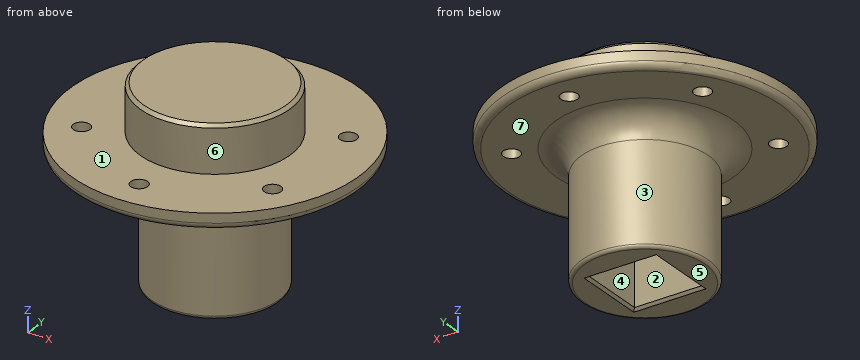
```python
from build123d import *

# Parameters (mm, degrees)
SKETCH1_R           = 20
BOSS_EXTRUDE1_DEPTH = 40
SKETCH2_W           = 21.283914114
SKETCH2_H           = 21.283914114
CUT_EXTRUDE1_DEPTH  = 15
CHAMFER1_SIZE       = 0.8
SKETCH3_R           = 45
BOSS_EXTRUDE2_DEPTH = 5
SKETCH4_R           = 23.5
BOSS_EXTRUDE3_DEPTH = 14.7
CHAMFER2_SIZE       = 1
FILLET1_R           = 2
FILLET2_R           = 8
SKETCH5_R           = 2.65
CUT_EXTRUDE2_DEPTH  = 78.942286398
CIRPATTERN1_COUNT   = 6
FILLET3_R           = 1


with BuildPart() as part:
    # Sketch1 → Boss-Extrude1 (new body)
    with BuildSketch(Plane.XY):
        Circle(SKETCH1_R)
    extrude(amount=BOSS_EXTRUDE1_DEPTH)

    # Sketch2 → Cut-Extrude1 (cut)
    with BuildSketch(Plane(origin=(0, 0, 0), x_dir=(-1, 0, 0), z_dir=(0, 0, -1))):
        Rectangle(SKETCH2_W, SKETCH2_H)
    extrude(amount=-CUT_EXTRUDE1_DEPTH, mode=Mode.SUBTRACT)

    # Chamfer1
    chamfer1_edges = [part.edges().sort_by_distance(p)[0] for p in [
        (0, -10.641957057, 0),
        (-10.641957057, 0, 0),
        (0, 10.641957057, 0),
        (10.641957057, 0, 0),
    ]]
    chamfer(chamfer1_edges, length=CHAMFER1_SIZE)

    # Sketch3 → Boss-Extrude2 (add)
    with BuildSketch(Plane.XY.offset(40)):
        Circle(SKETCH3_R)
    extrude(amount=BOSS_EXTRUDE2_DEPTH)

    # Sketch4 → Boss-Extrude3 (add)
    with BuildSketch(Plane.XY.offset(45)):
        Circle(SKETCH4_R)
    extrude(amount=BOSS_EXTRUDE3_DEPTH)

    # Chamfer2
    chamfer2_edges = [part.edges().sort_by_distance(p)[0] for p in [
        (-23.5, 0, 59.7),
    ]]
    chamfer(chamfer2_edges, length=CHAMFER2_SIZE)

    # Fillet1
    fillet1_edges = [part.edges().sort_by_distance(p)[0] for p in [
        (-45, 0, 40),
    ]]
    fillet(fillet1_edges, radius=FILLET1_R)

    # Fillet2
    fillet2_edges = [part.edges().sort_by_distance(p)[0] for p in [
        (-20, 0, 40),
    ]]
    fillet(fillet2_edges, radius=FILLET2_R)

    # Sketch5 → Cut-Extrude2 (cut, through all)
    with BuildSketch(Plane.XY.offset(45)):
        with Locations((0, 35)):
            Circle(SKETCH5_R)
    cut_extrude2 = extrude(amount=-CUT_EXTRUDE2_DEPTH, mode=Mode.SUBTRACT)

    # CirPattern1: Cut-Extrude2 ×6 about axis
    cirpattern1_axis = Axis((0, 0, 0), (0, 0, 1))
    for i in range(1, CIRPATTERN1_COUNT):
        add(cut_extrude2.rotate(cirpattern1_axis, i * 360 / CIRPATTERN1_COUNT), mode=Mode.SUBTRACT)

    # Fillet3
    fillet3_edges = [part.edges().sort_by_distance(p)[0] for p in [
        (-20, 0, 0),
    ]]
    fillet(fillet3_edges, radius=FILLET3_R)


solid = part.part
```
Geometry: final body of the model. Coordinates: model frame, mm. Face numbers are marked on the shaded views. A direction names the side the tool comes from. Round coordinates to 2 decimals unless told otherwise and drop trailing zeros. Write each loop counter-clockwise with the first axis right and the second up, starting at its lowest first coordinate (ties: lowest second). Pieces come first, ordered by that corner, then holes. Notation, with made-up numbers: (81, 38) -> (109, 38) arc R26 cw to (109, 65) -> close; hole circle Ø5 at (-19.5, -14). An arc over 180 degrees is marked (long way). Use CSV: the item, a comma, the result in double quotes. Start each with the question number.
Q1. Section A-A (x = 0). Give the number of separate pieces and of enclosed holes in the cut face, plus the area to 3 significant figures.
Q2. Line query: L1, parallel to Y at x = 0, z = 43.4; L2, parallel to Z at x = 9.5, y = 7; L3, parallel to Y at x = 0.5, z = 57.5. Output: solid intervals per line, ascending.
Q3. Section C-C (y = 0). Return loops of the section in (x, z), plus the area to 3 significant figures.
Q4. Section B-B (z = 10). Return loops of the section in (x, y), plus the area to 3 significant figures.
Q5. Reachability of the marked faces 5, 6 and 7 from +Z, -Z, +X, -X, +Y, -Y: full face, straight path, thin tool, end or side. Return the list, or none.
Q6. First-contact query: pin 1 Ø4.5 at (y, z) = (2, 9.5) entering from +X; pin 2 Ø11.5 at (x, z) = (-4.5, 10) entering from -Y; pin 3 Ø6 at (x, y) = (30.31, -17.5) entering from +Z. Flat tips, straight axial feed; report the tip coordinate or a pass-through.
Q7. Pull-direction query (Y, two-part tool) for the marked faces 1, 2, 3 and 4; classes: pulls with the +Y half, pulls with the -Y half, needs draft (parallel to the pull), parting line crosses it, or undercut.
Result sheet:
1,separate pieces,"3"
1,enclosed holes,"0"
1,area,"2,390 mm²"
2,L1,"-45 to -37.65, -32.35 to 32.35, 37.65 to 45"
2,L2,"15 to 59.7"
2,L3,"-23.49 to 23.49"
3,outline,"(-45, 42) arc R2 ccw to (-43, 40) -> (-28, 40) arc R8 cw to (-20, 32) -> (-20, 1) arc R1 ccw to (-19, 0) -> (-11.44, 0) -> (-10.64, 0.8) -> (-10.64, 15) -> (10.64, 15) -> (10.64, 0.8) -> (11.44, 0) -> (19, 0) arc R1 ccw to (20, 1) -> (20, 32) arc R8 cw to (28, 40) -> (43, 40) arc R2 ccw to (45, 42) -> (45, 45) -> (23.5, 45) -> (23.5, 58.7) -> (22.5, 59.7) -> (-22.5, 59.7) -> (-23.5, 58.7) -> (-23.5, 45) -> (-45, 45) -> close"
3,area,"2,450 mm²"
4,outline,"circle Ø40 at (0, 0); hole (-10.64, -10.64) -> (10.64, -10.64) -> (10.64, 10.64) -> (-10.64, 10.64) -> close"
4,area,"804 mm²"
5,face 5,"-Z, +X, -X, +Y, -Y"
5,face 6,"+Z"
5,face 7,"-Z"
6,pin 1,"x = 20"
6,pin 2,"y = -20"
6,pin 3,"z = 45"
7,face 1,"needs draft"
7,face 2,"undercut"
7,face 3,"parting line crosses it"
7,face 4,"undercut"
